from build123d import *

# Parameters (mm, degrees)
SKETCH1_W           = 12.7
SKETCH1_H           = 12.7
BOSS_EXTRUDE1_DEPTH = 2.54
FILLET1_R           = 0.635
SHELL1_START        = 0.635
SHELL1_OUTLINE_W    = 1.905
SHELL1_OUTLINE_H    = 11.43
SHELL1_DEPTH        = 11.43
SKETCH2_R           = 2.54
BOSS_EXTRUDE2_DEPTH = 1.905
SKETCH3_W           = 0.569871795
SKETCH3_H           = 3.175
BOSS_EXTRUDE3_DEPTH = 0.00254


# Read off the part's stored shape, not the designer's step: Shell1
with BuildPart() as part:
    # Sketch1 → Boss-Extrude1 (new body)
    with BuildSketch(Plane(origin=(0, 0, 0), x_dir=(1, 0, 0), z_dir=(0, 1, 0))):
        with Locations((6.35, 6.35)):
            Rectangle(SKETCH1_W, SKETCH1_H)
    extrude(amount=BOSS_EXTRUDE1_DEPTH)

    # Fillet1
    fillet1_edges = [part.edges().sort_by_distance(p)[0] for p in [
        (0, 1.27, -12.7),
        (12.7, 1.27, -12.7),
        (12.7, 1.27, 0),
        (0, 1.27, 0),
    ]]
    fillet(fillet1_edges, radius=FILLET1_R)

    # Shell1 outline → Shell1 (cut)
    with BuildSketch(Plane.YZ.offset(SHELL1_START)):
        with Locations((0.9525, -6.35)):
            Rectangle(SHELL1_OUTLINE_W, SHELL1_OUTLINE_H)
    extrude(amount=SHELL1_DEPTH, mode=Mode.SUBTRACT)

    # Sketch2 → Boss-Extrude2 (add)
    with BuildSketch(Plane(origin=(0, 1.905, 0), x_dir=(-1, 0, 0), z_dir=(0, -1, 0))):
        with Locations(Location((-6.35, 6.35, 0), (0, 0, 270))):
            Circle(SKETCH2_R)
    extrude(amount=BOSS_EXTRUDE2_DEPTH)

    # Sketch3 → Boss-Extrude3 (add)
    with BuildSketch(Plane(origin=(0, 2.54, 0), x_dir=(1, 0, 0), z_dir=(0, 1, 0))):
        with Locations((6.157871795, 6.4135)):
            Rectangle(SKETCH3_W, SKETCH3_H)
    extrude(amount=BOSS_EXTRUDE3_DEPTH)


solid = part.part
Design review of the part built by this model. Coordinates are the model's own, in mm. A direction names the side the tool comes from. Give positions to 0.01 mm unless a question says otherwise; leave off trailing zeros. Write each loop counter-clockwise with the first axis right and the second up, starting at its lowest first coordinate (ties: lowest second). Pieces come first, ordered by that corner, then holes. Notation, with made-up numbers: M 68.25,-8.75 L 93.25,-8.75 A15 ccw 93.25,0.25 Z; hole C 71.5,27.25 d11. An arc over 180 degrees is marked long. Return JSON: item names as keys, results as strings. Group by question number.
Item 1: The part is to be moulded in two halves that separate along Z. For faces 3 (the flat face through (0.635, 1, -6)), 4 (the flat face through (6, 0, -6)), 5 (the flat face through (6, 1, -12.7)), say which applies: pulls with the +Z half, pulls with the -Z half, needs draft (parallel to the pull), parting line crosses it, or undercut.
Item 2: Take a section at C-C (z = -2.25). Give the boundary of the cut face in (x, y) (3 decimals).
Item 3: Take a section at B-B (x = 3.5). Give the boundary of the cut face in (y, z) (3 decimals).
Item 4: Wall thickness on line 1 along Z through (x, y) = (2.5, 1.05) (3 decimals); line 2 along X through (y, z) = (1.4, -2.5) (3 decimals); line 3 along X through (y, z) = (0.1, -6) (3 decimals): over which ranges is each line inside the solid? List them lowest first.
Item 5: Clearance check with a flat-ended pin moving along its axis: pin 1 Ø2 at (x, z) = (10, -11) entering from -Y (3 decimals). State where the tip first meets the part, or that it passes through.
Item 6: Tool access review of faces 1 (the flat face through (0, 1, -6)), 2 (the flat face through (6, 1, -12.065)): name each direction out of +Z, -Z, +X, -X, +Y, -Y from which nothing blocks a thin tool from reaching the whole face with its end or side.
Return value:
{
 "1": {"face 3": "undercut", "face 4": "needs draft", "face 5": "pulls with the -Z half"},
 "2": {"outline": "M 0,0 L 0.635,0 L 0.635,1.905 L 12.065,1.905 L 12.065,0 L 12.7,0 L 12.7,2.54 L 0,2.54 Z"},
 "3": {"outline": "M 0,-12.7 L 2.54,-12.7 L 2.54,0 L 0,0 L 0,-0.635 L 1.905,-0.635 L 1.905,-12.065 L 0,-12.065 Z"},
 "4": {"line 1": "z = -12.7 to -12.065, -0.635 to 0", "line 2": "x = 0 to 0.635, 12.065 to 12.7", "line 3": "x = 0 to 0.635, 3.834 to 8.866, 12.065 to 12.7"},
 "5": {"pin 1": "stops at y = 1.905"},
 "6": {"face 1": "+Z, -Z, -X, +Y, -Y", "face 2": "-Y"}
}
